```python
from build123d import *

# Parameters (mm, degrees)
SKETCH_1_R      = 13.25
SKETCH_1_R_2    = 12.25
EXTRUDE_1_DEPTH = 7
SKETCH_2_R      = 13.25
SKETCH_2_R_2    = 8.5
EXTRUDE_2_DEPTH = 1
SKETCH_3_W      = 10
SKETCH_3_H      = 3
EXTRUDE_3_DEPTH = 3


with BuildPart() as part:
    # ｽｹｯﾁ1 → ﾎﾞｽ - 押し出し1 (new body)
    with BuildSketch(Plane.XY):
        Circle(SKETCH_1_R)
        Circle(SKETCH_1_R_2, mode=Mode.SUBTRACT)
    extrude(amount=EXTRUDE_1_DEPTH)

    # ｽｹｯﾁ2 → ﾎﾞｽ - 押し出し2 (add)
    with BuildSketch(Plane.XY.offset(7)):
        Circle(SKETCH_2_R)
        Circle(SKETCH_2_R_2, mode=Mode.SUBTRACT)
    extrude(amount=EXTRUDE_2_DEPTH)

    # ｽｹｯﾁ3 → ﾎﾞｽ - 押し出し3 (add)
    with BuildSketch(Plane.XY):
        with Locations((17.25, 1.556870996)):
            Rectangle(SKETCH_3_W, SKETCH_3_H)
    extrude(amount=EXTRUDE_3_DEPTH)


solid = part.part
```
Part model, mm, in its own coordinate system. A direction names the side the tool comes from. Round coordinates to 2 decimals unless told otherwise and drop trailing zeros. Order: outer loops, then holes, each group sorted by start corner. A loop starts at its lowest first (then second) coordinate and runs counter-clockwise, first axis right, second up. Notation, with made-up numbers: M -38,-31.5 L -13,-31.5 A24 cw -13,-0.5 Z; hole C 43.5,74.25 d10. An arc over 180 degrees is marked long. Put each result on its own line as item: value. Start each with the question number.
1. Drill centre lines: probe 1 along Y at (x, z) = (0, 7.75); probe 2 along Y at (x, z) = (0, 1.5); probe 3 along Z at (x, y) = (-5.5, -9). Where is each one in solid material? Low to high. Write a range as [from, to].
2. Slice it at A-A on x = 0. List the corners of the cut face in (y, z), then the cut area to 3 significant figures.
3. Slice it at B-B on z = 1. List the corners of the cut face in (x, y), then the cut area to 3 significant figures.
4. Tool access for faces 1 (the face through (2.6, 8.3, 7)), 2 (the face through (18, 0.057, 1)), 3 (the face through (18, 3.057, 1)): list every direction of +Z, -Z, +X, -X, +Y, -Y with a clear straight run to the whole face (end or side of a thin tool).
5. Drop flat-ended pins along their axis: pin 1 (0.9 mm diameter, centred on x = 17.5, z = 2, fed in from -Y); pin 2 (1.5 mm diameter, centred on x = 8, z = 6, fed in from -Y); pin 3 (1.5 mm diameter, centred on x = -7.5, y = 3, fed in from -Z). Give the stop position or say it passes through.
6. Slice it at D-D on x = 9.5. List the corners of the cut face in (y, z).
7. Slice it at C-C on y = 4. List the corners of the cut face in (x, z), then the cut area to 3 significant figures.
Findings:
1. probe 1: [-13.25, -8.5], [8.5, 13.25]
1. probe 2: [-13.25, -12.25], [12.25, 13.25]
1. probe 3: [7, 8]
2. outline: M -13.25,0 L -12.25,0 L -12.25,7 L -8.5,7 L -8.5,8 L -13.25,8 Z; M 8.5,7 L 12.25,7 L 12.25,0 L 13.25,0 L 13.25,8 L 8.5,8 Z
2. area: 23.5 mm2
3. outline: M 12.89,3.06 A13.25 ccw long 13.25,0.06 L 22.25,0.06 L 22.25,3.06 Z; hole C 0,0 d24.5
3. area: 107 mm2
4. face 1: -Z
4. face 2: +Z, -Z, +X, -Y
4. face 3: +Z, -Z, +X, +Y
5. pin 1: y = 0.06
5. pin 2: y = -11.09
5. pin 3: z = 7
6. outline: M -9.24,0 L -7.73,0 L -7.73,7 L 7.73,7 L 7.73,0 L 9.24,0 L 9.24,8 L -9.24,8 Z
7. outline: M -12.63,0 L -11.58,0 L -11.58,7 L -7.5,7 L -7.5,8 L -12.63,8 Z; M 7.5,7 L 11.58,7 L 11.58,0 L 12.63,0 L 12.63,8 L 7.5,8 Z
7. area: 25.0 mm2
